Geometry check sheet. Reference: the model listing, model coordinates, mm. Face numbers are marked on the shaded views. A direction names the side the tool comes from. Coordinates: 2 decimals unless noted, no trailing zeros. Loops run counter-clockwise (first coordinate to the right, second up) from the corner with the lowest first, then second, coordinate; pieces in that order, holes last.
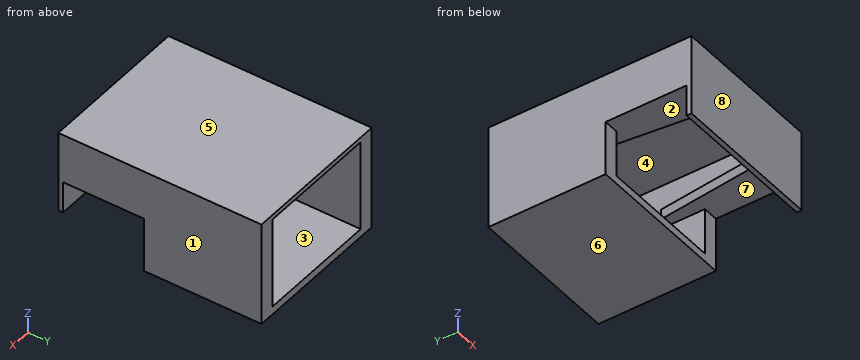
from build123d import *

# Parameters (mm, degrees)
SKETCH1_W           = 48.26
SKETCH1_H           = 25.4
BOSS_EXTRUDE1_DEPTH = 1.524
BOSS_EXTRUDE2_DEPTH = 36.83
SKETCH3_W           = 3.175
SKETCH3_H           = 3.175
BOSS_EXTRUDE3_DEPTH = 36.83
BOSS_EXTRUDE4_DEPTH = 3.175
SKETCH5_W           = 4.826
SKETCH5_H           = 11.43
BOSS_EXTRUDE5_DEPTH = 14.605
SKETCH7_W           = 2.54
SKETCH7_H           = 11.43
BOSS_EXTRUDE6_DEPTH = 48.26
SKETCH8_W           = 48.26
SKETCH8_H           = 32.639
SKETCH8_W_2         = 38.608
SKETCH8_H_2         = 28.575
BOSS_EXTRUDE7_DEPTH = 25.4


with BuildPart() as part:
    # Sketch1 → Boss-Extrude1 (new body)
    with BuildSketch(Plane(origin=(0, 0, 0), x_dir=(1, 0, 0), z_dir=(0, 1, 0))):
        with Locations((24.13, 12.7)):
            Rectangle(SKETCH1_W, SKETCH1_H)
    extrude(amount=BOSS_EXTRUDE1_DEPTH)

    # Sketch2 → Boss-Extrude2 (add)
    with BuildSketch(Plane(origin=(0, 1.524, 0), x_dir=(1, 0, 0), z_dir=(0, 1, 0))):
        Polygon((0, 15.494), (4.826, 15.494), (4.826, 1.524), (43.434, 1.524), (43.434, 15.494), (48.26, 15.494), (48.26, 0), (0, 0), align=None)
    extrude(amount=BOSS_EXTRUDE2_DEPTH)

    # Sketch3 → Boss-Extrude3 (add)
    with BuildSketch(Plane(origin=(0, 1.524, 0), x_dir=(1, 0, 0), z_dir=(0, 1, 0))):
        with Locations((6.4135, 13.9065)):
            Rectangle(SKETCH3_W, SKETCH3_H)
        with Locations((41.8465, 13.9065)):
            Rectangle(SKETCH3_W, SKETCH3_H)
    extrude(amount=BOSS_EXTRUDE3_DEPTH)

    # Sketch4 → Boss-Extrude4 (add)
    with BuildSketch(Plane(origin=(0, 0, -15.494), x_dir=(-1, 0, 0), z_dir=(0, 0, -1))):
        Polygon((-40.259, 38.354), (-36.195, 1.524), (-40.259, 1.524), align=None)
        Polygon((-8.001, 38.354), (-12.065, 1.524), (-8.001, 1.524), align=None)
    extrude(amount=-BOSS_EXTRUDE4_DEPTH)

    # Sketch5 → Boss-Extrude5 (add)
    with BuildSketch(Plane(origin=(0, 0, -15.494), x_dir=(-1, 0, 0), z_dir=(0, 0, -1))):
        with Locations((-45.847, 32.639)):
            Rectangle(SKETCH5_W, SKETCH5_H)
        with Locations((-2.413, 32.639)):
            Rectangle(SKETCH5_W, SKETCH5_H)
    extrude(amount=BOSS_EXTRUDE5_DEPTH)

    # Sketch7 → Boss-Extrude6 (add)
    with BuildSketch(Plane(origin=(48.26, 0, 0), x_dir=(0, 0, -1), z_dir=(1, 0, 0))):
        with Locations((31.369, 32.639)):
            Rectangle(SKETCH7_W, SKETCH7_H)
    extrude(amount=-BOSS_EXTRUDE6_DEPTH)

    # Sketch8 → Boss-Extrude7 (add)
    with BuildSketch(Plane(origin=(0, 38.354, 0), x_dir=(1, 0, 0), z_dir=(0, 1, 0))):
        with Locations((24.13, 16.3195)):
            Rectangle(SKETCH8_W, SKETCH8_H)
        with Locations((24.13, 15.8115)):
            Rectangle(SKETCH8_W_2, SKETCH8_H_2, mode=Mode.SUBTRACT)
    extrude(amount=BOSS_EXTRUDE7_DEPTH)


solid = part.part
1) Section check A-A on x = 26.5. Record the cut outline in (y, z), and give its area (3 significant figures).
Data:
outline: (0, -25.4) - (1.52, -25.4) - (1.52, -1.52) - (63.75, -1.52) - (63.75, 0) - (0, 0) - close; (26.92, -32.64) - (63.75, -32.64) - (63.75, -30.1) - (26.92, -30.1) - close
area: 227 mm2
2) Section check B-B on z = -19. Record the cut outline in (x, y).
Data:
outline: (0, 0) - (48.26, 0) - (48.26, 1.52) - (0, 1.52) - close; (0, 26.92) - (4.83, 26.92) - (4.83, 63.75) - (0, 63.75) - close; (43.43, 26.92) - (48.26, 26.92) - (48.26, 63.75) - (43.43, 63.75) - close
3) Depth check by flat-ended pin: pin 1 (19 mm diameter, centred on x = 32.5, z = -13.5, fed in from +Y); pin 2 (0.8 mm diameter, centred on x = 24, y = 0.5, fed in from -Z); pin 3 (13.5 mm diameter, centred on x = 7, y = 16, fed in from -Z). Enter the tip coordinate at first touch or a pass-through.
Data:
pin 1: stops at y = 38.35
pin 2: stops at z = -25.4
pin 3: stops at z = -15.49
4) Mould release check, pull along Z, two halves, no side actions. Record for the marked faces 5, 6, 7 and 8: +Z half, -Z half, draft (parallel to the pull), parting line (faces both ways), or undercut.
Data:
face 5: +Z half
face 6: -Z half
face 7: undercut
face 8: draft
5) Material ranges on probe 1 along Z at (x, y) = (7, 13); probe 2 along X at (y, z) = (57, -12.5); probe 3 along Y at (x, z) = (4, -21.5), recorded low to high.
Data:
probe 1: z = -15.49 to -12.32, -1.52 to 0
probe 2: x = 0 to 4.83, 43.43 to 48.26
probe 3: y = 0 to 1.52, 26.92 to 63.75
6) Access from +Z, -Z, +X, -X, +Y, -Y to the whole of each face (thin tool, end or side, straight path). Record for the marked faces 1, 2, 3 and 4.
Data:
face 1: +Z, -Z, +X, +Y, -Y
face 2: none
face 3: +Y, -Y
face 4: +Y
7) Section check D-D on z = -29. Record the cut outline in (x, y), and give its area (3 significant figures).
Data:
outline: (0, 26.92) - (4.83, 26.92) - (4.83, 63.75) - (0, 63.75) - close; (43.43, 26.92) - (48.26, 26.92) - (48.26, 63.75) - (43.43, 63.75) - close
area: 355 mm2
8) Section check C-C on y = 46. Record the cut outline in (x, z).
Data:
outline: (0, -32.64) - (48.26, -32.64) - (48.26, 0) - (0, 0) - close; hole (4.83, -30.1) - (43.43, -30.1) - (43.43, -1.52) - (4.83, -1.52) - close
